Read the model definition and answer for the solid it produces. Units are mm, in the model's axes. Coordinates: 2 decimals unless noted, no trailing zeros. Order: outer loops, then holes, each group sorted by start corner. A loop starts at its lowest first (then second) coordinate and runs counter-clockwise, first axis right, second up. Notation, with made-up numbers: (36, 67.5) - (59, 67.5) arc R34 cw to (59, 100.5) - close; hole circle Ø2 at (82, -30). An arc over 180 degrees is marked (long way). Use one line per item in the form item = value.
```python
from build123d import *

# Parameters (mm, degrees)
SKETCH1_W           = 35
SKETCH1_H           = 35
SKETCH1_R           = 7.45
SKETCH1_R_2         = 2
SKETCH1_R_3         = 2.5
BOSS_EXTRUDE1_DEPTH = 10


with BuildPart() as part:
    # Sketch1 → Boss-Extrude1 (new body)
    with BuildSketch(Plane.XY):
        with Locations((2.777777778, 2.470273614)):
            Rectangle(SKETCH1_W, SKETCH1_H)
        with Locations((2.777777778, 2.592592593)):
            Circle(SKETCH1_R, mode=Mode.SUBTRACT)
        with Locations((16.742243872, -11.49419248)):
            Circle(SKETCH1_R_2, mode=Mode.SUBTRACT)
        with Locations(Location((16.742243872, 16.434739708, 0), (0, 0, 180))):
            Circle(SKETCH1_R_2, mode=Mode.SUBTRACT)
        with Locations((-11.186688316, 16.434739708)):
            Circle(SKETCH1_R_2, mode=Mode.SUBTRACT)
        with Locations(Location((-11.186688316, -11.49419248, 0), (0, 0, 180))):
            Circle(SKETCH1_R_2, mode=Mode.SUBTRACT)
        with Locations(Location((15.277777778, 2.470273614, 0), (0, 0, 180))):
            Circle(SKETCH1_R_3, mode=Mode.SUBTRACT)
        with Locations((-9.722222222, 2.470273614)):
            Circle(SKETCH1_R_3, mode=Mode.SUBTRACT)
    extrude(amount=BOSS_EXTRUDE1_DEPTH)


solid = part.part
```
(1) Straight lines are drawn through the part: L1, parallel to X at y = 2, z = 6.25; L2, parallel to Y at x = -12, z = 3.5; L3, parallel to X at y = -10, z = 3.5. For each, find the intervals that lie inside material, in ascending order.
Answer list:
L1 = -14.72 to -12.18, -7.27 to -4.65, 10.2 to 12.82, 17.73 to 20.28
L2 = -15.03 to -13.32, -9.67 to 1.44, 3.5 to 14.61, 18.26 to 19.97
L3 = -14.72 to -12.52, -9.86 to 15.41, 18.07 to 20.28
(2) Section A-A, the plane x = 2 is taken. Write down the section's boundary in (y, z), then the cut area to 3 significant figures.
Answer list:
outline = (-15.03, 0) - (-4.82, 0) - (-4.82, 10) - (-15.03, 10) - close; (10, 0) - (19.97, 0) - (19.97, 10) - (10, 10) - close
area = 202 mm2
(3) Section D-D, the plane y = 8 is taken. Write down the section's boundary in (x, z), then the cut area to 3 significant figures.
Answer list:
outline = (-14.72, 0) - (-2.35, 0) - (-2.35, 10) - (-14.72, 10) - close; (7.9, 0) - (20.28, 0) - (20.28, 10) - (7.9, 10) - close
area = 248 mm2
(4) The mould has two halves that part along Y. Classify faces 1 (the flat face through (20.278, 2, 5)), 2 (the flat face through (3, -15.03, 5)), 3 (the cylindrical face through (-12.774, 15.218, 4.93)): +Y half, -Y half, draft (parallel to the pull), parting line (faces both ways), or undercut.
Answer list:
face_1 = draft
face_2 = -Y half
face_3 = undercut
(5) Section B-B, the plane z = 7 is taken. Write down the section's boundary in (x, y).
Answer list:
outline = (-14.72, -15.03) - (20.28, -15.03) - (20.28, 19.97) - (-14.72, 19.97) - close; hole circle Ø4 at (-11.19, -11.49); hole circle Ø4 at (-11.19, 16.43); hole circle Ø5 at (-9.72, 2.47); hole circle Ø14.9 at (2.78, 2.59); hole circle Ø5 at (15.28, 2.47); hole circle Ø4 at (16.74, -11.49); hole circle Ø4 at (16.74, 16.43)
(6) Section C-C, the plane y = 0.5 is taken. Write down the section's boundary in (x, z).
Answer list:
outline = (-14.72, 0) - (-11.26, 0) - (-11.26, 10) - (-14.72, 10) - close; (-8.18, 0) - (-4.37, 0) - (-4.37, 10) - (-8.18, 10) - close; (9.93, 0) - (13.74, 0) - (13.74, 10) - (9.93, 10) - close; (16.82, 0) - (20.28, 0) - (20.28, 10) - (16.82, 10) - close
